```python
from build123d import *

# Parameters (mm, degrees)
BOSS_EXTRUDE1_DEPTH  = 120
BOSS_EXTRUDE2_DEPTH  = 10
BOSS_EXTRUDE2_TAPER  = 45
SKETCH3_R            = 47.5
BOSS_EXTRUDE3_DEPTH  = 10
SKETCH4_R            = 42.5
BOSS_EXTRUDE4_DEPTH  = 35
SKETCH5_R            = 3.5
CUT_EXTRUDE1_DEPTH   = 10
BOSS_EXTRUDE5_DEPTH  = 110
SKETCH7_R            = 32.5
BOSS_EXTRUDE6_DEPTH  = 10
SKETCH8_R            = 32
BOSS_EXTRUDE7_DEPTH  = 11
SKETCH10_R           = 45
BOSS_EXTRUDE9_DEPTH  = 15.5
BOSS_EXTRUDE10_DEPTH = 65
SKETCH12_R           = 15
CUT_EXTRUDE2_DEPTH   = 20
SKETCH13_R           = 17.5
CUT_EXTRUDE3_DEPTH   = 22


with BuildPart() as part:
    # Sketch1 → Boss-Extrude1 (new body)
    with BuildSketch(Plane.XY):
        with BuildLine():
            Line((45, 60), (-45, 60))
            ThreePointArc((-45, 60), (-60.341439003, 0), (-45, -60))
            Line((-45, -60), (45, -60))
            ThreePointArc((45, -60), (60.341439003, 0), (45, 60))
        make_face()
    extrude(amount=BOSS_EXTRUDE1_DEPTH)

    # Sketch2 → Boss-Extrude2 (add)
    with BuildSketch(Plane.XY.offset(120)):
        with BuildLine():
            Line((45, 60), (-45, 60))
            ThreePointArc((-45, 60), (-60.341439003, 0), (-45, -60))
            Line((-45, -60), (45, -60))
            ThreePointArc((45, -60), (60.341439003, 0), (45, 60))
        make_face()
    extrude(amount=BOSS_EXTRUDE2_DEPTH, taper=BOSS_EXTRUDE2_TAPER)

    # Sketch3 → Boss-Extrude3 (add)
    with BuildSketch(Plane.XY.offset(130)):
        Circle(SKETCH3_R)
    extrude(amount=BOSS_EXTRUDE3_DEPTH)

    # Sketch4 → Boss-Extrude4 (add)
    with BuildSketch(Plane.XY.offset(140)):
        Circle(SKETCH4_R)
    extrude(amount=BOSS_EXTRUDE4_DEPTH)

    # Sketch5 → Cut-Extrude1 (cut)
    with BuildSketch(Plane.XY.offset(175)):
        with Locations((35, 0)):
            Circle(SKETCH5_R)
        with Locations(Location((0, 35, 0), (0, 0, 180))):
            Circle(SKETCH5_R)
        with Locations((30.310889132, 17.5)):
            Circle(SKETCH5_R)
        with Locations(Location((17.5, 30.310889132, 0), (0, 0, 180))):
            Circle(SKETCH5_R)
        with Locations(Location((30.310889132, -17.5, 0), (0, 0, 180))):
            Circle(SKETCH5_R)
        with Locations((17.5, -30.310889132)):
            Circle(SKETCH5_R)
        with Locations((0, -35)):
            Circle(SKETCH5_R)
        with Locations(Location((-17.5, -30.310889132, 0), (0, 0, 180))):
            Circle(SKETCH5_R)
        with Locations((-30.310889132, -17.5)):
            Circle(SKETCH5_R)
        with Locations(Location((-35, 0, 0), (0, 0, 180))):
            Circle(SKETCH5_R)
        with Locations(Location((-30.310889132, 17.5, 0), (0, 0, 180))):
            Circle(SKETCH5_R)
        with Locations((-17.5, 30.310889132)):
            Circle(SKETCH5_R)
    extrude(amount=-CUT_EXTRUDE1_DEPTH, mode=Mode.SUBTRACT)

    # Sketch6 → Boss-Extrude5 (add)
    with BuildSketch(Plane.XY.offset(175)):
        with BuildLine():
            Line((-20, -17), (-20, 17))
            ThreePointArc((-20, 17), (0, 25.404082058), (20, 17))
            Line((20, 17), (20, -17))
            ThreePointArc((20, -17), (0, -25.404082058), (-20, -17))
        make_face()
    extrude(amount=BOSS_EXTRUDE5_DEPTH)

    # Sketch7 → Boss-Extrude6 (add)
    with BuildSketch(Plane.XY.offset(285)):
        Circle(SKETCH7_R)
    extrude(amount=BOSS_EXTRUDE6_DEPTH)

    # Sketch8 → Boss-Extrude7 (add)
    with BuildSketch(Plane.XY.offset(295)):
        Circle(SKETCH8_R)
    extrude(amount=BOSS_EXTRUDE7_DEPTH)

    # Sketch10 → Boss-Extrude9 (add, symmetric)
    with BuildSketch(Plane.ZY.offset(45)):
        with Locations(Location((60, -60, 0), (0, 0, 180))):
            Circle(SKETCH10_R)
    extrude(amount=BOSS_EXTRUDE9_DEPTH, both=True)

    # Sketch11 → Boss-Extrude10 (add)
    with BuildSketch(Plane(origin=(-29.5, 0, 0), x_dir=(0, 0, -1), z_dir=(1, 0, 0))):
        with BuildLine():
            Line((-85, -60), (-35, -60))
            Line((-35, -60), (-35, -90))
            ThreePointArc((-35, -90), (-60, -100.505102572), (-85, -90))
            Line((-85, -90), (-85, -60))
        make_face()
    extrude(amount=BOSS_EXTRUDE10_DEPTH)

    # Sketch12 → Cut-Extrude2 (cut)
    with BuildSketch(Plane.XY.offset(306)):
        Circle(SKETCH12_R)
    extrude(amount=-CUT_EXTRUDE2_DEPTH, mode=Mode.SUBTRACT)

    # Sketch13 → Cut-Extrude3 (cut)
    with BuildSketch(Plane.ZY.offset(60.5)):
        with Locations(Location((60, -60, 0), (0, 0, 270))):
            Circle(SKETCH13_R)
    extrude(amount=-CUT_EXTRUDE3_DEPTH, mode=Mode.SUBTRACT)


solid = part.part
```
Geometry check sheet. Reference: the model listing, model coordinates, mm. A direction names the side the tool comes from. Give positions to 0.01 mm unless a question says otherwise; leave off trailing zeros. Loops run counter-clockwise (first coordinate to the right, second up) from the corner with the lowest first, then second, coordinate; pieces in that order, holes last. Notation, with made-up numbers: M 84,72 L 96,72 A17 cw 96,76 Z; hole C 29,2.25 d4. An arc over 180 degrees is marked long. Write item = value, one per line.
(1) Sectioned sample at B-B, the plane z = 30. Record the cut outline in (x, y).
Answer below:
outline = M -60.5,-93.54 L -29.5,-93.54 L -29.5,-60 L 45,-60 A125 ccw 45,60 L -45,60 A125 ccw -57.51,-26.46 L -60.5,-26.46 Z
(2) Sectioned sample at A-A, the plane z = 82. Record the cut outline in (x, y).
Answer below:
outline = M -60.5,-99.26 L -29.5,-99.26 L -29.5,-92.73 L 35.5,-92.73 L 35.5,-60 L 45,-60 A125 ccw 45,60 L -45,60 A125 ccw -58.61,-20.74 L -60.5,-20.74 Z
(3) Gauge pin test, flat ends, axial feed: pin 1 Ø4 at (y, z) = (-11.5, 55.5) entering from -X; pin 2 Ø10 at (x, y) = (43, -21.5) entering from +Z; pin 3 Ø4 at (x, y) = (17.5, -30.31) entering from +Z. Record the tip position at first contact, or that the pin passes through.
Answer below:
pin_1 = -59.98
pin_2 = 140
pin_3 = 165
(4) Tool access check on faces 1 (the face through (3, -75, 85)), 2 (the face through (-0.312, 25.402, 229.23)), 3 (the face through (0.312, -25.402, 229.23)), 4 (the face through (19.115, -33.416, 170.07)). Record the directions out of +Z, -Z, +X, -X, +Y, -Y that give a thin tool (end or side, any length) a straight path to the whole face; none if there is none.
Answer below:
face_1 = +Z, +X, -Y
face_2 = +Y
face_3 = -Y
face_4 = none
(5) Release check for a two-part mould opening along Z. For faces 5 (the face through (2.545, -100.503, 59.61)), 6 (the face through (-33.727, -25.861, 157.255)), 7 (the face through (-33.808, -17.346, 170.07)) record: released by +Z, released by -Z, zero draft, split by the parting line, or undercut.
Answer below:
face_5 = split by the parting line
face_6 = zero draft
face_7 = undercut
(6) Material ranges on line 1 (Y direction, x = 0, z = 168); line 2 (Z direction, x = -31.5, y = -43.5); line 3 (Y direction, x = 0, z = 293), recorded low to high. Write a range as [from, to].
Answer below:
line_1 = [-42.5, -38.5], [-31.5, 31.5], [38.5, 42.5]
line_2 = [0, 130]
line_3 = [-32.5, -15], [15, 32.5]
